from build123d import *

# Parameters (mm, degrees)
SKETCH1_R           = 2.4892
SKETCH1_R_2         = 2.37186857
BOSS_EXTRUDE1_DEPTH = 2.286
CUT_EXTRUDE1_DEPTH  = 819.47149982
FILLET1_R           = 5.08


with BuildPart() as part:
    # Sketch1 → Boss-Extrude1 (new body)
    with BuildSketch(Plane.XY):
        with BuildLine():
            Line((238.806714439, 781.287169191), (222.296714439, 781.287169191))
            Line((222.296714439, 781.287169191), (176.576714439, 781.287169191))
            Line((176.576714439, 781.287169191), (116.886714439, 781.287169191))
            ThreePointArc((116.886714439, 781.287169191), (113.29461199, 779.799271639), (111.806714439, 776.207169191))
            Line((111.806714439, 776.207169191), (111.806714439, 757.885949725))
            ThreePointArc((111.806714439, 757.885949725), (112.159468576, 756.025964093), (113.16874064, 754.424292487))
            Line((113.16874064, 754.424292487), (162.347850631, 701.603741569))
            ThreePointArc((162.347850631, 701.603741569), (175.968112644, 666.987169191), (162.347850631, 632.370596813))
            Line((162.347850631, 632.370596813), (113.16874064, 579.550045895))
            ThreePointArc((113.16874064, 579.550045895), (112.159468576, 577.948374289), (111.806714439, 576.088388657))
            Line((111.806714439, 576.088388657), (111.806714439, 557.767169191))
            ThreePointArc((111.806714439, 557.767169191), (113.29461199, 554.175066742), (116.886714439, 552.687169191))
            Line((116.886714439, 552.687169191), (176.576714439, 552.687169191))
            Line((176.576714439, 552.687169191), (222.296714439, 552.687169191))
            Line((222.296714439, 552.687169191), (238.806714439, 552.687169191))
            ThreePointArc((238.806714439, 552.687169191), (242.398816887, 554.175066742), (243.886714439, 557.767169191))
            Line((243.886714439, 557.767169191), (243.886714439, 666.987169191))
            Line((243.886714439, 666.987169191), (243.886714439, 776.207169191))
            ThreePointArc((243.886714439, 776.207169191), (242.398816887, 779.799271639), (238.806714439, 781.287169191))
        make_face()
        with Locations((142.286714439, 768.587169191)):
            Circle(SKETCH1_R, mode=Mode.SUBTRACT)
        with Locations((154.986714439, 768.587169191)):
            Circle(SKETCH1_R, mode=Mode.SUBTRACT)
        with Locations((167.686714439, 768.587169191)):
            Circle(SKETCH1_R, mode=Mode.SUBTRACT)
        with Locations((231.186714439, 743.187169191)):
            Circle(SKETCH1_R_2, mode=Mode.SUBTRACT)
        with Locations((231.186714439, 730.487169191)):
            Circle(SKETCH1_R, mode=Mode.SUBTRACT)
        with Locations((231.186714439, 717.787169191)):
            Circle(SKETCH1_R, mode=Mode.SUBTRACT)
        with Locations((231.186714439, 705.087169191)):
            Circle(SKETCH1_R, mode=Mode.SUBTRACT)
        with Locations((231.186714439, 692.387169191)):
            Circle(SKETCH1_R, mode=Mode.SUBTRACT)
        with Locations(Location((167.686714439, 565.387169191, 0), (0, 0, 180))):
            Circle(SKETCH1_R, mode=Mode.SUBTRACT)
        with Locations(Location((154.986714439, 565.387169191, 0), (0, 0, 180))):
            Circle(SKETCH1_R, mode=Mode.SUBTRACT)
        with Locations(Location((142.286714439, 565.387169191, 0), (0, 0, 180))):
            Circle(SKETCH1_R, mode=Mode.SUBTRACT)
        with Locations((231.186714439, 616.187169191)):
            Circle(SKETCH1_R, mode=Mode.SUBTRACT)
        with Locations((231.186714439, 603.487169191)):
            Circle(SKETCH1_R, mode=Mode.SUBTRACT)
        with Locations((231.186714439, 590.787169191)):
            Circle(SKETCH1_R, mode=Mode.SUBTRACT)
        with Locations((231.186714439, 565.387169191)):
            Circle(SKETCH1_R, mode=Mode.SUBTRACT)
        with Locations(Location((231.186714439, 768.587169191, 0), (0, 0, 180))):
            Circle(SKETCH1_R, mode=Mode.SUBTRACT)
        with Locations((231.186714439, 654.287169191)):
            Circle(SKETCH1_R, mode=Mode.SUBTRACT)
        with Locations((231.186714439, 641.587169191)):
            Circle(SKETCH1_R, mode=Mode.SUBTRACT)
        with Locations((231.186714439, 628.887169191)):
            Circle(SKETCH1_R, mode=Mode.SUBTRACT)
        with Locations((116.886714439, 768.587169191)):
            Circle(SKETCH1_R, mode=Mode.SUBTRACT)
        with Locations((129.586714439, 768.587169191)):
            Circle(SKETCH1_R, mode=Mode.SUBTRACT)
        with Locations((129.586714439, 565.387169191)):
            Circle(SKETCH1_R, mode=Mode.SUBTRACT)
        with Locations((116.886714439, 565.387169191)):
            Circle(SKETCH1_R, mode=Mode.SUBTRACT)
        with Locations((231.186714439, 679.687169191)):
            Circle(SKETCH1_R, mode=Mode.SUBTRACT)
        with Locations((231.186714439, 666.987169191)):
            Circle(SKETCH1_R, mode=Mode.SUBTRACT)
        with Locations((231.186714439, 755.887169191)):
            Circle(SKETCH1_R_2, mode=Mode.SUBTRACT)
        with Locations((231.186714439, 578.087169191)):
            Circle(SKETCH1_R, mode=Mode.SUBTRACT)
        with Locations(Location((180.386714439, 565.387169191, 0), (0, 0, 180))):
            Circle(SKETCH1_R, mode=Mode.SUBTRACT)
        with Locations(Location((193.086714439, 565.387169191, 0), (0, 0, 180))):
            Circle(SKETCH1_R, mode=Mode.SUBTRACT)
        with Locations(Location((205.786714439, 565.387169191, 0), (0, 0, 180))):
            Circle(SKETCH1_R, mode=Mode.SUBTRACT)
        with Locations(Location((218.486714439, 565.387169191, 0), (0, 0, 180))):
            Circle(SKETCH1_R, mode=Mode.SUBTRACT)
        with Locations((180.386714439, 768.587169191)):
            Circle(SKETCH1_R, mode=Mode.SUBTRACT)
        with Locations((193.086714439, 768.587169191)):
            Circle(SKETCH1_R, mode=Mode.SUBTRACT)
        with Locations((205.786714439, 768.587169191)):
            Circle(SKETCH1_R, mode=Mode.SUBTRACT)
        with Locations((218.486714439, 768.587169191)):
            Circle(SKETCH1_R, mode=Mode.SUBTRACT)
        with BuildLine():
            Line((150.786953537, 728.930511953), (170.473797978, 707.785965632))
            ThreePointArc((170.473797978, 707.785965632), (174.010528598, 706.170857078), (177.653429014, 707.529649071))
            Line((177.653429014, 707.529649071), (200.363611972, 728.674195392))
            ThreePointArc((200.363611972, 728.674195392), (201.629200597, 734.252154823), (196.901954734, 737.472169191))
            Line((196.901954734, 737.472169191), (154.504927335, 737.472169191))
            ThreePointArc((154.504927335, 737.472169191), (149.847051276, 734.419628344), (150.786953537, 728.930511953))
        make_face(mode=Mode.SUBTRACT)
        with BuildLine():
            Line((213.406714439, 674.585176614), (213.406714439, 722.206352957))
            ThreePointArc((213.406714439, 722.206352957), (210.354173591, 726.864229016), (204.865057201, 725.924326755))
            Line((204.865057201, 725.924326755), (181.115086252, 703.811675273))
            ThreePointArc((181.115086252, 703.811675273), (179.499977697, 700.274944652), (180.858769691, 696.632044236))
            Line((180.858769691, 696.632044236), (204.60874064, 671.123519376))
            ThreePointArc((204.60874064, 671.123519376), (210.186700071, 669.857930751), (213.406714439, 674.585176614))
        make_face(mode=Mode.SUBTRACT)
        with BuildLine():
            Line((180.858769691, 637.342294146), (204.60874064, 662.850819006))
            ThreePointArc((204.60874064, 662.850819006), (210.186700071, 664.116407631), (213.406714439, 659.389161768))
            Line((213.406714439, 659.389161768), (213.406714439, 611.767985425))
            ThreePointArc((213.406714439, 611.767985425), (210.354173591, 607.110109366), (204.865057201, 608.050011626))
            Line((204.865057201, 608.050011626), (181.115086252, 630.162663109))
            ThreePointArc((181.115086252, 630.162663109), (179.499977697, 633.699393729), (180.858769691, 637.342294146))
        make_face(mode=Mode.SUBTRACT)
        with BuildLine():
            Line((200.363611972, 605.30014299), (177.653429014, 626.44468931))
            ThreePointArc((177.653429014, 626.44468931), (174.010528598, 627.803481304), (170.473797978, 626.188372749))
            Line((170.473797978, 626.188372749), (150.786953537, 605.043826429))
            ThreePointArc((150.786953537, 605.043826429), (149.847051276, 599.554710038), (154.504927335, 596.502169191))
            Line((154.504927335, 596.502169191), (196.901954734, 596.502169191))
            ThreePointArc((196.901954734, 596.502169191), (201.629200597, 599.722183559), (200.363611972, 605.30014299))
        make_face(mode=Mode.SUBTRACT)
    extrude(amount=BOSS_EXTRUDE1_DEPTH)

    # Sketch3 → Cut-Extrude1 (cut, through all)
    with BuildSketch(Plane.XY.offset(2.286)):
        with BuildLine():
            Line((243.886714439, 557.767169191), (243.886714439, 560.307169191))
            Line((243.886714439, 560.307169191), (111.806714439, 560.307169191))
            Line((111.806714439, 560.307169191), (111.806714439, 557.767169191))
            ThreePointArc((111.806714439, 557.767169191), (113.29461199, 554.175066742), (116.886714439, 552.687169191))
            Line((116.886714439, 552.687169191), (238.806714439, 552.687169191))
            ThreePointArc((238.806714439, 552.687169191), (242.398816887, 554.175066742), (243.886714439, 557.767169191))
        make_face()
        with BuildLine():
            Line((111.806714439, 776.207169191), (111.806714439, 773.667169191))
            Line((111.806714439, 773.667169191), (243.886714439, 773.667169191))
            Line((243.886714439, 773.667169191), (243.886714439, 776.207169191))
            ThreePointArc((243.886714439, 776.207169191), (242.398816887, 779.799271639), (238.806714439, 781.287169191))
            Line((238.806714439, 781.287169191), (116.886714439, 781.287169191))
            ThreePointArc((116.886714439, 781.287169191), (113.29461199, 779.799271639), (111.806714439, 776.207169191))
        make_face()
    extrude(amount=-CUT_EXTRUDE1_DEPTH, mode=Mode.SUBTRACT)

    # Fillet1
    fillet1_edges = [part.edges().sort_by_distance(p)[0] for p in [
        (111.806714439, 560.307169191, 1.143),
        (243.886714439, 560.307169191, 1.143),
        (243.886714439, 773.667169191, 1.143),
        (111.806714439, 773.667169191, 1.143),
    ]]
    fillet(fillet1_edges, radius=FILLET1_R)


solid = part.part
Could you check a few things on this model? Use its own coordinates, in mm. A direction names the side the tool comes from. Coordinates: 2 decimals unless noted, no trailing zeros. Order: outer loops, then holes, each group sorted by start corner. A loop starts at its lowest first (then second) coordinate and runs counter-clockwise, first axis right, second up. Notation, with made-up numbers: (57, -34.75) -> (110, -34.75) arc R20 cw to (110, -1.75) -> close; hole circle Ø7 at (57, -13.75). An arc over 180 degrees is marked (long way). One line per item, written item: value. Start each with the question number.
1) If I drill on L1, parallel to Y at x = 128, z = 0.35; L2, parallel to Y at x = 212.5, z = 2; L3, parallel to X at y = 641, z = 0.85, over which ranges is the centre line in solid material (lowest first)? Write a range as [from, to].
2) We'd pull the mould along Y, two halves only. Please class faces 3 (the cylindrical face through (205.247, 766.157, 1.127)), 4 (the cylindrical face through (242.438, 561.835, 1.127)), 5 (the cylindrical face through (193.41, 562.92, 1.13)), 6 (the flat face through (192, 668, 2.286)): +Y half, -Y half, draft (parallel to the pull), parting line (faces both ways), or undercut.
3) Which directions (+Z, -Z, +X, -X, +Y, -Y) give clear straight access to the entire face, cutting with the end or side of a thin tool? Please do faces 1 (the flat face through (192.568, 684.056, 1.127)), 2 (the cylindrical face through (175.965, 667.52, 1.127)).
4) Imagine slicing it at B-B on x = 193.5. List the corners of the cut face in (y, z) for me.
5) Imagine slicing it at A-A on x = 124. List the corners of the cut face in (y, z) for me.
6) Imagine slicing it at C-C on z = 1.9. Count the separate pieces of the cut face and the enclosed holes in it, plus the area to 3 significant figures.
Answer list:
1. L1: y = [560.31, 563.47], [567.31, 595.48], [738.49, 766.67], [770.51, 773.67]
1. L2: y = [560.31, 608.87], [662.29, 671.69], [725.1, 773.67]
1. L3: x = [168.82, 184.26], [213.41, 228.77], [233.61, 243.89]
2. face 3: undercut
2. face 4: -Y half
2. face 5: undercut
2. face 6: draft
3. face 1: +Z, -Z
3. face 2: +Z, -Z, -X
4. outline: (560.31, 0) -> (562.93, 0) -> (562.93, 2.29) -> (560.31, 2.29) -> close; (567.84, 0) -> (596.5, 0) -> (596.5, 2.29) -> (567.84, 2.29) -> close; (611.69, 0) -> (618.63, 0) -> (618.63, 2.29) -> (611.69, 2.29) -> close; (650.92, 0) -> (683.05, 0) -> (683.05, 2.29) -> (650.92, 2.29) -> close; (715.34, 0) -> (722.28, 0) -> (722.28, 2.29) -> (715.34, 2.29) -> close; (737.47, 0) -> (766.13, 0) -> (766.13, 2.29) -> (737.47, 2.29) -> close; (771.04, 0) -> (773.67, 0) -> (773.67, 2.29) -> (771.04, 2.29) -> close
5. outline: (560.31, 0) -> (591.18, 0) -> (591.18, 2.29) -> (560.31, 2.29) -> close; (742.79, 0) -> (773.67, 0) -> (773.67, 2.29) -> (742.79, 2.29) -> close
6. separate pieces: 1
6. enclosed holes: 39
6. area: 16,000 mm2
